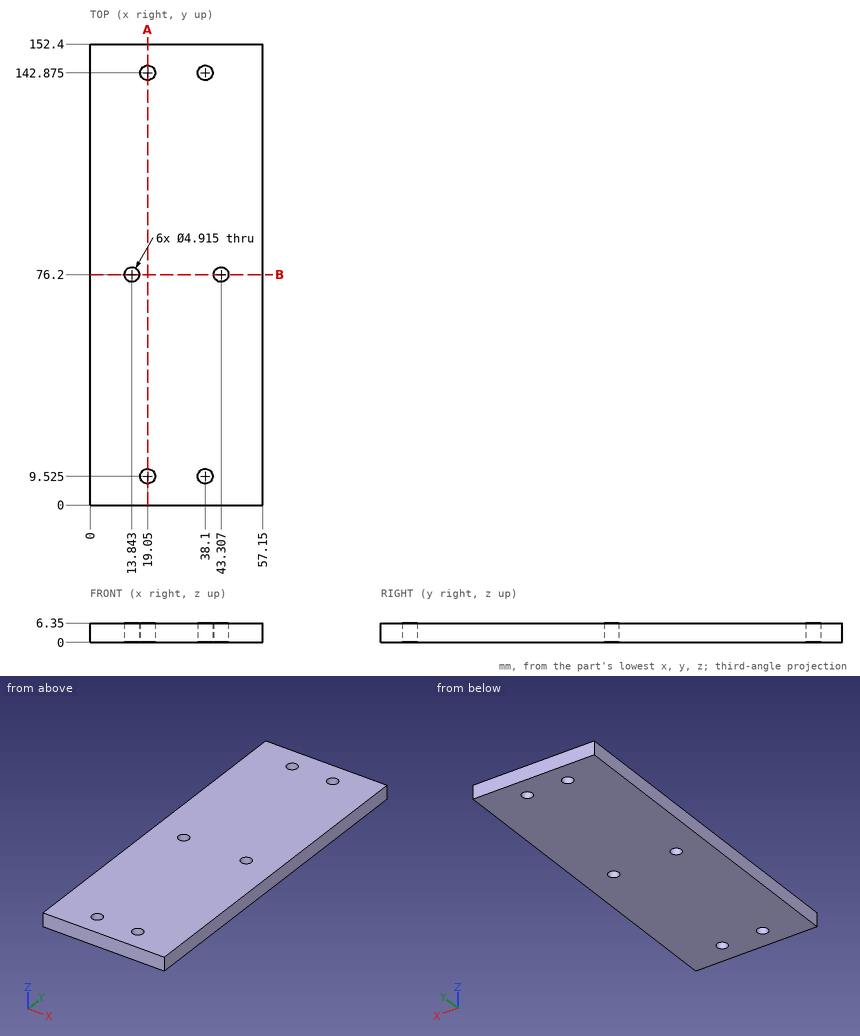
Geometry: see drawing. Coordinates: mm, zero at the bounding-box minimum. Coordinates: 2 decimals unless noted, no trailing zeros. Loops run counter-clockwise (first coordinate to the right, second up) from the corner with the lowest first, then second, coordinate; pieces in that order, holes last. Notation, with made-up numbers: M 20,43 L 53,43 A6 cw 53,53 Z; hole C -30,13 d5. An arc over 180 degrees is marked long. Put each result on its own line as item: value. Start each with the question number.
1) Cut plane A-A on x = 19.05. Return the cut outline in (y, z).
2) Cut plane B-B on y = 76.2. Return the cut outline in (x, z), then the cut area to 4 significant figures.
3) Ray query, L1, parallel to X at y = 143, z = 5.25; L2, parallel to X at y = 142.5, z = 5; L3, parallel to Y at x = 38, z = 3.75. Return the intervals inside material, ascending. Write a range as from..to.
The answers:
1. outline: M 0,0 L 7.07,0 L 7.07,6.35 L 0,6.35 Z; M 11.98,0 L 140.42,0 L 140.42,6.35 L 11.98,6.35 Z; M 145.33,0 L 152.4,0 L 152.4,6.35 L 145.33,6.35 Z
2. outline: M 0,0 L 11.39,0 L 11.39,6.35 L 0,6.35 Z; M 16.3,0 L 40.85,0 L 40.85,6.35 L 16.3,6.35 Z; M 45.76,0 L 57.15,0 L 57.15,6.35 L 45.76,6.35 Z
2. area: 300.5 mm²
3. L1: x = 0..16.6, 21.5..35.65, 40.55..57.15
3. L2: x = 0..16.62, 21.48..35.67, 40.53..57.15
3. L3: y = 0..7.07, 11.98..140.42, 145.33..152.4
